from build123d import *

# Parameters (mm, degrees)
SKETCH5_W      = 49.45
SKETCH5_H      = 49.45
SKETCH5_W_2    = 43.1
SKETCH5_H_2    = 43.1
EXTRUDE1_DEPTH = 4.8
SKETCH6_R      = 1.5
SKETCH6_R_2    = 2.38125
SKETCH6_R_3    = 11.2
EXTRUDE2_DEPTH = 6.5
SKETCH7_R      = 6
EXTRUDE3_DEPTH = 4.5
SKETCH8_R      = 6
EXTRUDE4_DEPTH = 3.5
SKETCH9_R      = 15.3625
EXTRUDE5_DEPTH = 3


with BuildPart() as part:
    # Sketch5 → Extrude1 (new body)
    with BuildSketch(Plane.XY):
        with Locations((-46.55, 0)):
            Rectangle(SKETCH5_W, SKETCH5_H)
        with Locations((-46.55, 0)):
            Rectangle(SKETCH5_W_2, SKETCH5_H_2, mode=Mode.SUBTRACT)
    extrude(amount=EXTRUDE1_DEPTH)

    # Sketch6 → Extrude2 (add)
    with BuildSketch(Plane(origin=(0, 0, 0), x_dir=(-1, 0, 0), z_dir=(0, 0, -1))):
        Polygon((8.45, 38.1), (8.45, -37.987007671), (84.65, -38.1), (84.65, 38.1), align=None)
        with Locations((62.05, 15.5)):
            Circle(SKETCH6_R, mode=Mode.SUBTRACT)
        with Locations((31.05, 15.5)):
            Circle(SKETCH6_R, mode=Mode.SUBTRACT)
        with Locations((62.05, -15.5)):
            Circle(SKETCH6_R, mode=Mode.SUBTRACT)
        with Locations((31.05, -15.5)):
            Circle(SKETCH6_R, mode=Mode.SUBTRACT)
        with Locations((14.17, 32.38)):
            Circle(SKETCH6_R_2, mode=Mode.SUBTRACT)
        with Locations((78.93, 32.38)):
            Circle(SKETCH6_R_2, mode=Mode.SUBTRACT)
        with Locations((78.93, -33.309394929)):
            Circle(SKETCH6_R_2, mode=Mode.SUBTRACT)
        with Locations((14.17, -32.38)):
            Circle(SKETCH6_R_2, mode=Mode.SUBTRACT)
        with Locations((46.55, 0)):
            Circle(SKETCH6_R_3, mode=Mode.SUBTRACT)
    extrude(amount=EXTRUDE2_DEPTH)

    # Sketch7 → Extrude3 (cut)
    with BuildSketch(Plane(origin=(0, 0, -6.5), x_dir=(-1, 0, 0), z_dir=(0, 0, -1))):
        with Locations((62.05, -15.5)):
            Circle(SKETCH7_R)
        with Locations((31.05, -15.5)):
            Circle(SKETCH7_R)
    extrude(amount=-EXTRUDE3_DEPTH, mode=Mode.SUBTRACT)

    # Sketch8 → Extrude4 (cut)
    with BuildSketch(Plane(origin=(0, 0, -6.5), x_dir=(-1, 0, 0), z_dir=(0, 0, -1))):
        with Locations((62.05, 15.5)):
            Circle(SKETCH8_R)
        with Locations((31.05, 15.5)):
            Circle(SKETCH8_R)
    extrude(amount=-EXTRUDE4_DEPTH, mode=Mode.SUBTRACT)

    # Sketch9 → Extrude5 (cut)
    with BuildSketch(Plane(origin=(0, 0, -6.5), x_dir=(-1, 0, 0), z_dir=(0, 0, -1))):
        with Locations((46.55, 0)):
            Circle(SKETCH9_R)
    extrude(amount=-EXTRUDE5_DEPTH, mode=Mode.SUBTRACT)


solid = part.part
Input: part model. Units: mm. Frame: model coordinates. A direction names the side the tool comes from. Round coordinates to 2 decimals unless told otherwise and drop trailing zeros. Order: outer loops, then holes, each group sorted by start corner. A loop starts at its lowest first (then second) coordinate and runs counter-clockwise, first axis right, second up. Notation, with made-up numbers: (68, 84) - (111, 84) arc R26 ccw to (111, 111) - close; hole circle Ø2 at (-30.5, 44). An arc over 180 degrees is marked (long way). Answer as a JSON object with one key per item and string values. Group by question number.
(1) Pin query (flat end, axial travel): P1, Ø1.8, axis at x = -62.05, y = -15.5, coming from the -Z side; P2, Ø3.5, axis at x = -64, y = 18.5, coming from the -Z side; P3, Ø1.5, axis at y = 12.5, z = 1, coming from the -X side (3 decimals); P4, Ø1.4, axis at y = 4.5, z = 2.5, coming from the +X side (3 decimals). Return the tip coordinate at first contact, or that it passes through.
(2) Cut plane D-D (x = -78.93). Return loops of the section in (y, z), then the cut area to 3 significant figures.
(3) Cut plane B-B (x = -46.5). Return loops of the section in (y, z) (3 decimals).
(4) Draft query along X for faces 4 (the face through (-8.45, 1, -3)), 5 (the face through (-32.48, 15.95, -1.48)), 6 (the face through (-46, 17, -6.5)), 7 (the face through (-63, -17, -2)). Return one class per face: released by +X, released by -X, zero draft, split by the parting line, or undercut.
(5) Material intervals for probe 1 along Y at (x, z) = (-78.93, -4); probe 2 along X at (y, z) = (15.5, -2.2); probe 3 along X at (y, z) = (17, 3) (3 decimals), sorted ascending. Write a range as from..to.
(6) Cut plane C-C (z = 3.25). Return loops of the section in (x, y) (3 decimals), then the cut area to 3 significant figures.
(7) Reachability of faces 1 (the face through (-57.63, -11.44, -4.28)), 2 (the face through (-47, -21.55, 2)), 3 (the face through (-76.55, -33.2, -3.2)) from +Z, -Z, +X, -X, +Y, -Y: full face, straight path, thin tool, end or side. Return the list, or none.
Here are the results:
{
 "1": {"P1": "passes through", "P2": "stops at z = -3", "P3": "stops at x = -71.275", "P4": "stops at x = -21.825"},
 "2": {"outline": "(-38.09, -6.5) - (-35.69, -6.5) - (-35.69, 0) - (-38.09, 0) - close; (-30.93, -6.5) - (30, -6.5) - (30, 0) - (-30.93, 0) - close; (34.76, -6.5) - (38.1, -6.5) - (38.1, 0) - (34.76, 0) - close", "area": "433 mm^2"},
 "3": {"outline": "(-38.043, -6.5) - (-15.362, -6.5) - (-15.362, -3.5) - (-11.2, -3.5) - (-11.2, 0) - (-21.55, 0) - (-21.55, 4.8) - (-24.725, 4.8) - (-24.725, 0) - (-38.043, 0) - close; (11.2, -3.5) - (15.362, -3.5) - (15.362, -6.5) - (38.1, -6.5) - (38.1, 0) - (24.725, 0) - (24.725, 4.8) - (21.55, 4.8) - (21.55, 0) - (11.2, 0) - close"},
 "4": {"face 4": "released by +X", "face 5": "undercut", "face 6": "zero draft", "face 7": "undercut"},
 "5": {"probe 1": "y = -38.09..-35.69, -30.93..30, 34.76..38.1", "probe 2": "x = -84.65..-63.55, -60.55..-32.55, -29.55..-8.45", "probe 3": "x = -71.275..-68.1, -25..-21.825"},
 "6": {"outline": "(-71.275, -24.725) - (-21.825, -24.725) - (-21.825, 24.725) - (-71.275, 24.725) - close; hole (-68.1, -21.55) - (-25, -21.55) - (-25, 21.55) - (-68.1, 21.55) - close", "area": "588 mm^2"},
 "7": {"face 1": "-Z", "face 2": "+Z", "face 3": "+Z, -Z"}
}
